The model under review builds one solid part; all positions refer to its coordinate system, in mm. Give positions to 0.01 mm unless a question says otherwise; leave off trailing zeros. Loops run counter-clockwise (first coordinate to the right, second up) from the corner with the lowest first, then second, coordinate; pieces in that order, holes last. Notation, with made-up numbers: (22.5, -25) -> (73.5, -25) arc R9 cw to (73.5, -8) -> close; hole circle Ø6 at (87.25, -24.5). An arc over 180 degrees is marked (long way). Write each question's results on one line, items separated by ' | '. Start each with the question number.
Q1. Wall thickness on L1, parallel to Z at x = 0, y = 50.5; L2, parallel to X at y = -26, z = 0: over which ranges is each line inside the solid? List them lowest first. Write a range as [from, to].
Q2. We need section D-D (y = -11.5). Write out the cut boundary in (x, z), plus the area to 3 significant figures.
Q3. We need section B-B (y = 91.5). Write out the cut boundary in (x, z).
Q4. Insertion check: pin 1 Ø12 at (x, y) = (-13, 128.5) entering from +Z; pin 2 Ø5 at (y, z) = (36.5, -2) entering from +X; pin 3 Ø24 at (x, z) = (0, 0) entering from +Y; pin 4 Ø10 at (y, z) = (40.5, -13.5) entering from +X. Each pin has a flat end and moves straight along its axis. Give the tip position at first contact, or say it passes through.
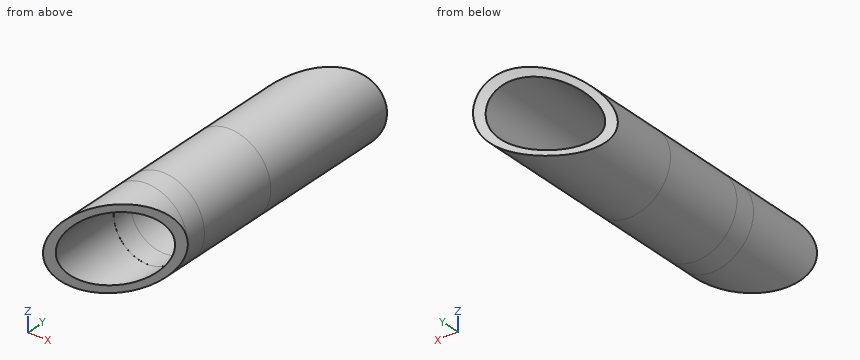
Autodesk Inventor part; units mm, degrees
ref_plane "Work Plane4" through (15.0868, 167.4868, 0) normal (0.7071068, 0.7071068, 0) x (0, 0, -1)
ref_plane "Work Plane5" through (0, 0, 0) normal (-0.7071068, -0.7071068, 0) x (0, 0, -1)
ref_plane "Work Plane6" through (0, 0, 0) normal (-0.7071068, -0.7071068, 0) x (0, 0, -1)
sketch "Sketch1" plane through (0, 0, 0) normal (0, 1, 0) x (-1, 0, 0)
  circle A0 centre (0, 0) radius 20.066
  circle A1 centre (0, 0) radius 24.2951
  dimension "d0" = 40.132
  dimension "d1" = 48.5902
extrude "Extrusion1" add sketch "Sketch1" along normal blind 152.4
ref_plane "Work Plane4" through (15.0868, 167.4868, 0) normal (0.7071068, 0.7071068, 0) x (0, 0, -1)
ref_plane "Work Plane3" through (0, 152.4, 0) normal (0.7071068, 0.7071068, 0) x (0, 0, -1)
sketch "Sketch2" plane through (15.0868, 167.4868, 0) normal (0.7071068, 0.7071068, 0) x (0, 0, -1)
  ellipse E0 centre (0, 0) end of major axis (24.2951, 0) minor radius 17.1792
  line L0 (0, -17.1792) -> (46.559, -17.1792)
  line L1 (0, -17.1792) -> (-63.5901, -17.1792)
  line L2 (0, -17.1792) -> (0, 39.92)
  line L3 (0, 39.92) -> (57.0992, 39.92)
  arc A0 (-57.0992, 39.92) -> (57.0992, 39.92) centre (0, 39.92) ccw
  line L4 (57.0992, 39.92) -> (-57.0992, 39.92)
  point P0 (0, -107.7631)
  dimension "d6" = 57.0992
  dimension "d7" = 57.0992
  dimension "d8" = 114.1984
extrude "Extrusion2" cut sketch "Sketch2" against normal blind 152.4
sketch "Sketch3" plane through (0, 0, 0) normal (0, -1, 0) x (1, 0, 0)
  circle A0 centre (0, 0) radius 77.6216
extrude "Extrusion3" cut sketch "Sketch3" against normal blind 63.5
sketch "Sketch4" plane through (0, 63.5, 0) normal (0, -1, 0) x (1, 0, 0)
  circle A0 centre (0, 0) radius 20.066
  circle A1 centre (0, 0) radius 24.2951
extrude "Extrusion4" add sketch "Sketch4" along normal blind 50.8
sketch "Sketch5" plane through (0, 12.7, 0) normal (0, -1, 0) x (1, 0, 0)
  circle A0 centre (0, 0) radius 19.9816
  circle A1 centre (0, 0) radius 24.2951
extrude "Extrusion5" add sketch "Sketch5" along normal blind 12.7
ref_plane "Work Plane5" through (0, 0, 0) normal (-0.7071068, -0.7071068, 0) x (0, 0, -1)
ref_plane "Work Plane6" through (0, 0, 0) normal (-0.7071068, -0.7071068, 0) x (0, 0, -1)
ref_plane "Work Plane9" through (12.1413, -12.1413, 0) normal (0.7071068, -0.7071068, 0) x (0, 0, 1)
ref_plane "Work Plane8" through (-12.1413, 12.1413, 0) normal (0.7071068, -0.7071068, 0) x (0, 0, 1)
sketch "Sketch6" plane through (0, 0, 0) normal (0, -1, 0) x (1, 0, 0)
  circle A0 centre (0, 0) radius 20.0088
  circle A1 centre (0, 0) radius 24.2951
extrude "Extrusion6" add sketch "Sketch6" along normal blind 50.8
sketch "Sketch7" plane through (12.1413, -12.1413, 0) normal (0.7071068, -0.7071068, 0) x (0, 0, 1)
  line L0 (26.0117, 61.2493) -> (-25.7555, 61.2493)
  line L1 (-25.7555, 61.2493) -> (-25.7555, -22.8083)
  line L2 (-25.7555, -22.8083) -> (26.0117, -22.8083)
  line L3 (26.0117, -22.8083) -> (26.0117, 61.2493)
  point P0 (0, 0)
extrude "Extrusion7" cut sketch "Sketch7" along normal blind 50.8
ref_plane "Work Plane1" through (0, 76.2, 0) normal (0, 1, 0) x (1, 0, 0)
ref_plane "Work Plane2" through (0, 152.4, 0) normal (0, 1, 0) x (1, 0, 0)
ref_plane "Work Plane7" through (0, 0, 0) normal (0.7071068, -0.7071068, 0) x (0, 0, 1)
properties part number "Angled Pipe (Attached to Control Pipe)"
Output:
1) L1: [-24.3, -20.07], [20.07, 24.3] | L2: [-24.3, -20.01]
2) outline: (12.78, -20.66) -> (12.78, -15.4) arc R20.01 cw (long way) to (12.78, 15.4) -> (12.78, 20.66) arc R24.3 ccw (long way) to start | area: 415 mm2
3) outline: circle Ø48.59 at (0, 0); hole circle Ø40.13 at (0, 0)
4) pin 1: z = 23.26 | pin 2: x = 24.3 | pin 3: through | pin 4: x = 22.76
